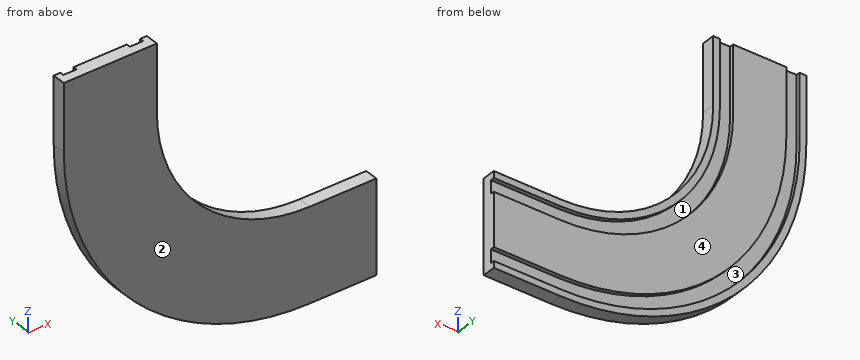
from build123d import *

# Parameters (mm, degrees)
BOSS_EXTRUDE1_DEPTH = 10
CUT_SWEEP1_START    = 7
CUT_SWEEP1_DEPTH    = 3


# Read off the part's stored shape, not the designer's step: Cut-Sweep1
with BuildPart() as part:
    # Sketch1 → Boss-Extrude1 (new body)
    with BuildSketch(Plane(origin=(0, 0, 0), x_dir=(1, 0, 0), z_dir=(0, 1, 0))):
        with BuildLine():
            Line((-35, 0), (35, 0))
            Line((35, 0), (35, 50))
            ThreePointArc((35, 50), (68.682720164, 131.317279836), (150, 165))
            Line((150, 165), (200, 165))
            Line((200, 165), (200, 235))
            Line((200, 235), (150, 235))
            ThreePointArc((150, 235), (19.18524548, 180.81475452), (-35, 50))
            Line((-35, 50), (-35, 0))
        make_face()
    extrude(amount=BOSS_EXTRUDE1_DEPTH)

    # Cut-Sweep1 outline → Cut-Sweep1 (cut)
    with BuildSketch(Plane(origin=(0, 0, 0), x_dir=(1, 0, 0), z_dir=(0, 1, 0)).offset(CUT_SWEEP1_START)):
        with BuildLine():
            Line((-30, 50), (-30, 0))
            Line((-30, 0), (-20, 0))
            Line((-20, 0), (-20, 50))
            ThreePointArc((-20, 50), (29.791847198, 170.208152802), (150, 220))
            Line((150, 220), (200, 220))
            Line((200, 220), (200, 230))
            Line((200, 230), (150, 230))
            ThreePointArc((150, 230), (22.720779386, 177.279220614), (-30, 50))
        make_face()
        with BuildLine():
            Line((20, 50), (20, 0))
            Line((20, 0), (30, 0))
            Line((30, 0), (30, 50))
            ThreePointArc((30, 50), (65.147186258, 134.852813742), (150, 170))
            Line((150, 170), (200, 170))
            Line((200, 170), (200, 180))
            Line((200, 180), (150, 180))
            ThreePointArc((150, 180), (58.076118446, 141.923881554), (20, 50))
        make_face()
    extrude(amount=CUT_SWEEP1_DEPTH, mode=Mode.SUBTRACT)


solid = part.part
Model file for the job. Use its own axes, mm. Face numbers are marked on the shaded views. A direction names the side the tool comes from. Round coordinates to 2 decimals unless told otherwise and drop trailing zeros. Loops run counter-clockwise (first coordinate to the right, second up) from the corner with the lowest first, then second, coordinate; pieces in that order, holes last.
1. Tool access for the marked faces 1 and 2: list every direction of +Z, -Z, +X, -X, +Y, -Y with a clear straight run to the whole face (end or side of a thin tool).
Check values:
face 1: +Y
face 2: +Z, -Z, +X, -X, -Y
2. Drop flat-ended pins along their axis: P1, Ø0.9, axis at x = 169.5, y = 8, coming from the +Z side; P2, Ø6, axis at y = 2.5, z = -135, coming from the -X side; P3, Ø0.9, axis at y = 8, z = -19, coming from the +X side. Give the stop position or say it passes through.
Check values:
P1: stops at z = -165
P2: stops at x = -15.83
P3: stops at x = 35
3. Band-saw the part on A-A, the plane z = -43. List the corners of the cut face in (x, y).
Check values:
outline: (-35, 0) - (35, 0) - (35, 10) - (30, 10) - (30, 7) - (20, 7) - (20, 10) - (-20, 10) - (-20, 7) - (-30, 7) - (-30, 10) - (-35, 10) - close
4. Band-saw the part on B-B, the plane x = 165. List the corners of the cut face in (y, z).
Check values:
outline: (0, -235) - (10, -235) - (10, -230) - (7, -230) - (7, -220) - (10, -220) - (10, -180) - (7, -180) - (7, -170) - (10, -170) - (10, -165) - (0, -165) - close
5. Mould opens along Z. For the marked faces 3 and 4 say: +Z half, -Z half, draft (parallel to the pull), parting line (faces both ways), or undercut.
Check values:
face 3: undercut
face 4: draft
6. Wall check: probe 1 along Z at (x, y) = (157.5, 9.25); probe 2 along X at (y, z) = (9.25, -67); probe 3 along Z at (x, y) = (79.5, 9.25). Give the ranges that are in metal, low to high.
Check values:
probe 1: z = -235 to -230, -220 to -180, -170 to -165
probe 2: x = -34.22 to -29.2, -19.15 to 21.12, 31.21 to 36.26
probe 3: z = -221.04 to -215.62, -204.69 to -159.22, -147.11 to -140.86
7. Band-saw the part on C-C, the plane y = 1.5. List the corners of the cut face in (x, z).
Check values:
outline: (-35, -50) arc R185 ccw to (150, -235) - (200, -235) - (200, -165) - (150, -165) arc R115 cw to (35, -50) - (35, 0) - (-35, 0) - close
